Read the model definition and answer for the solid it produces. Units are mm, in the model's axes. A direction names the side the tool comes from. Coordinates: 2 decimals unless noted, no trailing zeros. Write each loop counter-clockwise with the first axis right and the second up, starting at its lowest first coordinate (ties: lowest second). Pieces come first, ordered by that corner, then holes. Notation, with made-up numbers: (80, 39) -> (94, 39) arc R20 ccw to (94, 78) -> close; hole circle Ø7 at (39, 70.25). An arc over 180 degrees is marked (long way). One line per item, written item: value. Start each with the question number.
1. For a pull along Y with two mould halves and no side action, classify faces 1 (the flat face through (13, 10.16, -13)), 2 (the cylindrical face through (12.15, -1.25, -15.18)), 3 (the flat face through (10, 2.54, -16)) as pulls with the +Y half, pulls with the -Y half, needs draft (parallel to the pull), parting line crosses it, or undercut.
2. For faces 4 (the flat face through (25.4, 1, -13)), 5 (the cylindrical face through (9.68, 6.3, -10.38)), 6 (the cylindrical face through (10.18, 11.45, -10.77)), determine the directions among +Z, -Z, +X, -X, +Y, -Y from which every point of the face is accessible in a straight line to the end or side of a thin tool.
3. Consider line 1 along Y through (x, z) = (20.25, -16.25); line 2 along Z through (x, y) = (12.7, 11.6) (3 decimals); line 3 along X through (y, z) = (11.25, -12.7) (3 decimals). Determine where each line is inside the solid, lowest interval first.
4. Given P1, Ø5, axis at x = 7.5, z = -14, coming from the -Y side; P2, Ø1, axis at x = 12, y = 4, coming from the +Z side; P3, Ø3, axis at y = 8, z = -19, coming from the +X side, each flat-ended and moving along its own axis, determine where each tip first touches the part or whether it passes through.
5. Find section C-C, the plane x = 2.75. Write down the section's boundary in (y, z), and give its area (3 significant figures).
6. Find section A-A, the plane z = -21.25. Write down the section's boundary in (x, y), and give its area (3 significant figures).
7. Find section D-D, the plane y = 8.75. Write down the section's boundary in (x, z), and give its area (3 significant figures).
8. Find section B-B, the plane x = 12.7. Write down the section's boundary in (y, z) (3 decimals), and give its area (3 significant figures).
```python
from build123d import *

# Parameters (mm, degrees)
SKETCH1_W           = 25.4
SKETCH1_H           = 25.4
BOSS_EXTRUDE1_DEPTH = 2.54
SKETCH2_R           = 2.54
BOSS_EXTRUDE2_DEPTH = 2.54
SKETCH3_R           = 3.81
BOSS_EXTRUDE3_DEPTH = 7.62
SKETCH4_W           = 25.4
SKETCH4_H           = 25.4
BOSS_EXTRUDE4_DEPTH = 2.54
SKETCH5_R           = 3.175
CUT_EXTRUDE2_DEPTH  = 2.54


with BuildPart() as part:
    # Sketch1 → Boss-Extrude1 (new body)
    with BuildSketch(Plane(origin=(0, 0, 0), x_dir=(1, 0, 0), z_dir=(0, 1, 0))):
        with Locations((12.7, 12.7)):
            Rectangle(SKETCH1_W, SKETCH1_H)
    extrude(amount=BOSS_EXTRUDE1_DEPTH)

    # Sketch2 → Boss-Extrude2 (add)
    with BuildSketch(Plane.XZ):
        with Locations((12.7, -12.7)):
            Circle(SKETCH2_R)
    extrude(amount=BOSS_EXTRUDE2_DEPTH)

    # Sketch3 → Boss-Extrude3 (add)
    with BuildSketch(Plane(origin=(0, 2.54, 0), x_dir=(1, 0, 0), z_dir=(0, 1, 0))):
        with Locations((12.7, 12.7)):
            Circle(SKETCH3_R)
    extrude(amount=BOSS_EXTRUDE3_DEPTH)

    # Sketch4 → Boss-Extrude4 (add)
    with BuildSketch(Plane(origin=(0, 10.16, 0), x_dir=(1, 0, 0), z_dir=(0, 1, 0))):
        with Locations((12.7, 12.7)):
            Rectangle(SKETCH4_W, SKETCH4_H)
    extrude(amount=BOSS_EXTRUDE4_DEPTH)

    # Sketch5 → Cut-Extrude2 (cut)
    with BuildSketch(Plane(origin=(0, 12.7, 0), x_dir=(1, 0, 0), z_dir=(0, 1, 0))):
        with Locations((12.7, 12.7)):
            Circle(SKETCH5_R)
    extrude(amount=-CUT_EXTRUDE2_DEPTH, mode=Mode.SUBTRACT)


solid = part.part
```
Answer block:
1. face 1: pulls with the +Y half
1. face 2: needs draft
1. face 3: undercut
2. face 4: +Z, -Z, +X, +Y, -Y
2. face 5: none
2. face 6: +Y
3. line 1: y = 0 to 2.54, 10.16 to 12.7
3. line 2: z = -25.4 to -15.875, -9.525 to 0
3. line 3: x = 0 to 9.525, 15.875 to 25.4
4. P1: stops at y = 0
4. P2: stops at z = -8.9
4. P3: passes through
5. outline: (0, -25.4) -> (2.54, -25.4) -> (2.54, 0) -> (0, 0) -> close; (10.16, -25.4) -> (12.7, -25.4) -> (12.7, 0) -> (10.16, 0) -> close
5. area: 129 mm2
6. outline: (0, 0) -> (25.4, 0) -> (25.4, 2.54) -> (0, 2.54) -> close; (0, 10.16) -> (25.4, 10.16) -> (25.4, 12.7) -> (0, 12.7) -> close
6. area: 129 mm2
7. outline: circle Ø7.62 at (12.7, -12.7)
7. area: 45.6 mm2
8. outline: (-2.54, -15.24) -> (0, -15.24) -> (0, -25.4) -> (2.54, -25.4) -> (2.54, -16.51) -> (10.16, -16.51) -> (10.16, -25.4) -> (12.7, -25.4) -> (12.7, -15.875) -> (10.16, -15.875) -> (10.16, -9.525) -> (12.7, -9.525) -> (12.7, 0) -> (10.16, 0) -> (10.16, -8.89) -> (2.54, -8.89) -> (2.54, 0) -> (0, 0) -> (0, -10.16) -> (-2.54, -10.16) -> close
8. area: 184 mm2
